Read the model definition and answer for the solid it produces. Units are mm, in the model's axes. Round coordinates to 2 decimals unless told otherwise and drop trailing zeros. Order: outer loops, then holes, each group sorted by start corner. A loop starts at its lowest first (then second) coordinate and runs counter-clockwise, first axis right, second up. Notation, with made-up numbers: (85.5, 73) - (116.5, 73) arc R29 ccw to (116.5, 107) - close; hole circle Ø1 at (60, -8.75). An arc over 180 degrees is marked (long way). Answer as a JSON object with one key per item and string values. Group by question number.
Q1. A cutting plane is placed at D-D on y = -1.75. Determine the outline of the cut face in (x, z).
Q2. Consider line 1 (Y direction, x = 0, z = 17.6); line 2 (Z direction, x = -0.4, y = 0.7); line 3 (Y direction, x = -0.1, z = 1.5). Determine where each line is inside the solid, lowest interval first.
Q3. A cutting plane is placed at A-A on x = 0. Determine the outline of the cut face in (y, z), and give its area (3 significant figures).
Q4. Given pin 1 Ø1 at (y, z) = (0.5, 5.5) entering from -X; pin 2 Ø0.9 at (y, z) = (-2, 5.5) entering from +X; pin 3 Ø0.9 at (y, z) = (-2, 7) entering from -X, each flat-ended and moving along its own axis, determine where each tip first touches the part or whether it passes through.
Q5. A cutting plane is placed at C-C on z = 10. Determine the outline of the cut face in (x, y), and give its area (3 significant figures).
Q6. A cutting plane is placed at B-B on y = 0. Determine the outline of the cut face in (x, z).
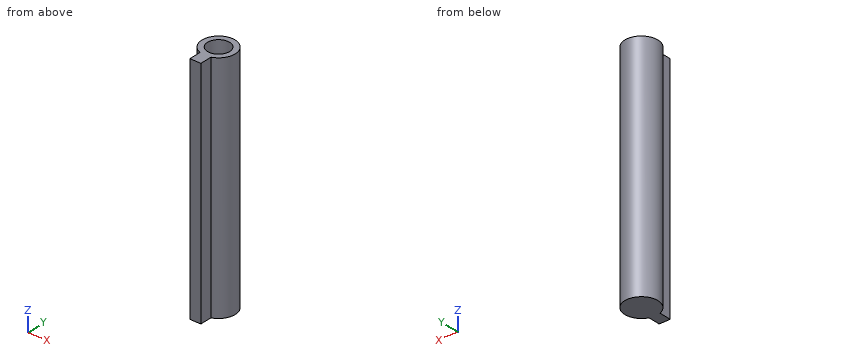
```python
from build123d import *

# Parameters (mm, degrees)
SKETCH1_R               = 5
BOSS_EXTRUDE1_DEPTH     = 21
CUT_EXTRUDE1_DEPTH      = 23.158519806
CUT_EXTRUDE1_DEPTH_BACK = 23.158519806
SKETCH2_OUTSIDE_W       = 17.064
SKETCH2_OUTSIDE_H       = 17.064
SKETCH6_R               = 1
CUT_EXTRUDE4_DEPTH      = 6


with BuildPart() as part:
    # Sketch1 → Boss-Extrude1 (new body)
    with BuildSketch(Plane.XY):
        with Locations(Location((0, 0, 0), (0, 0, 180))):
            Circle(SKETCH1_R)
    extrude(amount=BOSS_EXTRUDE1_DEPTH)

    # Sketch2 outside → Cut-Extrude1 (cut, two sides: drawn at the far end of the back side and taken through both)
    with BuildSketch(Plane(origin=(0, 0, 0), x_dir=(-1, 0, 0), z_dir=(0, 0, -1)).offset(-CUT_EXTRUDE1_DEPTH_BACK)):
        Rectangle(SKETCH2_OUTSIDE_W, SKETCH2_OUTSIDE_H)
        with BuildLine():
            Line((-0.5, -1.414213562), (-0.5, -2.514213562))
            Line((-0.5, -2.514213562), (0.5, -2.514213562))
            Line((0.5, -2.514213562), (0.5, -1.414213562))
            ThreePointArc((0.5, -1.414213562), (0, 1.5), (-0.5, -1.414213562))
        make_face(mode=Mode.SUBTRACT)
    extrude(amount=CUT_EXTRUDE1_DEPTH + CUT_EXTRUDE1_DEPTH_BACK, mode=Mode.SUBTRACT)

    # Sketch6 → Cut-Extrude4 (cut)
    with BuildSketch(Plane.XY.offset(21)):
        Circle(SKETCH6_R)
    extrude(amount=-CUT_EXTRUDE4_DEPTH, mode=Mode.SUBTRACT)


solid = part.part
```
Result set:
{
 "1": {"outline": "(-0.5, 0) - (0.5, 0) - (0.5, 21) - (-0.5, 21) - close"},
 "2": {"line 1": "y = -2.51 to -1, 1 to 1.5", "line 2": "z = 0 to 15", "line 3": "y = -2.51 to 1.5"},
 "3": {"outline": "(-2.51, 0) - (1.5, 0) - (1.5, 21) - (1, 21) - (1, 15) - (-1, 15) - (-1, 21) - (-2.51, 21) - close", "area": "72.3 mm²"},
 "4": {"pin 1": "stops at x = -1.5", "pin 2": "stops at x = 0.5", "pin 3": "stops at x = -0.5"},
 "5": {"outline": "(-0.5, -2.51) - (0.5, -2.51) - (0.5, -1.41) arc R1.5 ccw (long way) to (-0.5, -1.41) - close", "area": "8.11 mm²"},
 "6": {"outline": "(-1.5, 0) - (1.5, 0) - (1.5, 21) - (1, 21) - (1, 15) - (-1, 15) - (-1, 21) - (-1.5, 21) - close"}
}
